Can you work these out from the model? Positions are in its coordinate system, mm. A direction names the side the tool comes from. Coordinates: 2 decimals unless noted, no trailing zeros. Order: outer loops, then holes, each group sorted by start corner. A loop starts at its lowest first (then second) coordinate and runs counter-clockwise, first axis right, second up.
```python
from build123d import *

# Parameters (mm, degrees)
SKETCH1_W              = 220
SKETCH1_H              = 90
SKETCH1_R              = 3
SKETCH1_R_2            = 5.25
BOSS_EXTRUDE1_DEPTH    = 4
SKETCH3_W              = 4
SKETCH3_H              = 90
BOSS_EXTRUDE2_DEPTH    = 10
SKETCH21_W             = 220
SKETCH21_H             = 90
SKETCH21_R             = 5.25
SKETCH21_R_2           = 10
SKETCH21_R_3           = 5
BOSS_EXTRUDE3_DEPTH    = 4
CUT_EXTRUDE4_REACH     = 240.109
SKETCH35_R             = 5
BOSS_EXTRUDE6_DEPTH    = 4
SKETCH33_W             = 1
SKETCH33_H             = 43.95
CUT_EXTRUDE2_DEPTH     = 4
CUT_EXTRUDE3_DEPTH     = 4
SKETCH41_W             = 4
SKETCH41_H             = 16
BOSS_EXTRUDE8_DEPTH    = 26
CONVERT_SOLID4_DEPTH   = 90
CONVERT_SOLID4_START   = 13
CONVERT_SOLID4_2_DEPTH = 20
CONVERT_SOLID4_3_DEPTH = 2
CONVERT_SOLID4_START_2 = 31
CONVERT_SOLID4_4_DEPTH = 2
CONVERT_SOLID4_5_DEPTH = 90
CONVERT_SOLID4_START_3 = 15
CONVERT_SOLID4_6_DEPTH = 16


# Read off the part's stored shape, not the designer's step: Convert-Solid4
with BuildPart() as part:
    # Sketch1 → Boss-Extrude1 (new body)
    with BuildSketch(Plane.XY):
        with Locations((110, 45)):
            Rectangle(SKETCH1_W, SKETCH1_H)
        with Locations((201, 44.75)):
            Circle(SKETCH1_R, mode=Mode.SUBTRACT)
        with Locations((201, 77.75)):
            Circle(SKETCH1_R_2, mode=Mode.SUBTRACT)
        with Locations((15, 44.75)):
            Circle(SKETCH1_R, mode=Mode.SUBTRACT)
        with Locations((15, 77.75)):
            Circle(SKETCH1_R_2, mode=Mode.SUBTRACT)
    extrude(amount=BOSS_EXTRUDE1_DEPTH)

    # Sketch3 → Boss-Extrude2 (add)
    with BuildSketch(Plane.XY.offset(4)):
        with Locations((2, 45)):
            Rectangle(SKETCH3_W, SKETCH3_H)
        with Locations((218, 45)):
            Rectangle(SKETCH3_W, SKETCH3_H)
    extrude(amount=BOSS_EXTRUDE2_DEPTH)

    # Sketch21 → Boss-Extrude3 (add)
    with BuildSketch(Plane.XY.offset(14)):
        with Locations((110, 45)):
            Rectangle(SKETCH21_W, SKETCH21_H)
        with Locations((201, 77.75)):
            Circle(SKETCH21_R, mode=Mode.SUBTRACT)
        with Locations((15, 77.75)):
            Circle(SKETCH21_R, mode=Mode.SUBTRACT)
        with Locations((15, 44.75)):
            Circle(SKETCH21_R_2, mode=Mode.SUBTRACT)
        with Locations((201, 44.75)):
            Circle(SKETCH21_R_2, mode=Mode.SUBTRACT)
        with Locations((100, 20)):
            Circle(SKETCH21_R_3, mode=Mode.SUBTRACT)
        with Locations((173.090932683, 46.602923891)):
            Circle(SKETCH21_R_3, mode=Mode.SUBTRACT)
        with Locations((155, 75)):
            Circle(SKETCH21_R_3, mode=Mode.SUBTRACT)
    extrude(amount=BOSS_EXTRUDE3_DEPTH)

    # Sketch35 → Cut-Extrude4 (cut, up to next)
    with BuildSketch(Plane.XY.offset(4), mode=Mode.PRIVATE) as cut_extrude4_sk1:
        with Locations((100, 20)):
            Circle(SKETCH35_R)
    cut_extrude4_tool1 = extrude(cut_extrude4_sk1.sketch, amount=-CUT_EXTRUDE4_REACH, mode=Mode.PRIVATE) & part.part
    # Sketch35 → Cut-Extrude4 (cut, up to next)
    with BuildSketch(Plane.XY.offset(4), mode=Mode.PRIVATE) as cut_extrude4_sk2:
        with Locations((173.090932683, 46.602923891)):
            Circle(SKETCH35_R)
    cut_extrude4_tool2 = extrude(cut_extrude4_sk2.sketch, amount=-CUT_EXTRUDE4_REACH, mode=Mode.PRIVATE) & part.part
    # Sketch35 → Cut-Extrude4 (cut, up to next)
    with BuildSketch(Plane.XY.offset(4), mode=Mode.PRIVATE) as cut_extrude4_sk3:
        with Locations((155, 75)):
            Circle(SKETCH35_R)
    cut_extrude4_tool3 = extrude(cut_extrude4_sk3.sketch, amount=-CUT_EXTRUDE4_REACH, mode=Mode.PRIVATE) & part.part
    add(cut_extrude4_tool1.solids().sort_by_distance((100, 20, 4))[0], mode=Mode.SUBTRACT)
    add(cut_extrude4_tool2.solids().sort_by_distance((173.090933, 46.602924, 4))[0], mode=Mode.SUBTRACT)
    add(cut_extrude4_tool3.solids().sort_by_distance((155, 75, 4))[0], mode=Mode.SUBTRACT)

    # Sketch24 → Boss-Extrude6 (add)
    with BuildSketch(Plane(origin=(220, 0, 0), x_dir=(0, 0, -1), z_dir=(1, 0, 0))):
        with BuildLine():
            Line((40, 42.05), (40, 46.05))
            Line((40, 46.05), (0, 46.05))
            Line((0, 46.05), (0, 0))
            Line((0, 0), (40, 0))
            Line((40, 0), (40, 3.95))
            Line((40, 3.95), (35, 3.95))
            ThreePointArc((35, 3.95), (25.715537172, 6.365660518), (18.785731592, 13))
            Line((18.785731592, 13), (15.95, 13))
            Line((15.95, 13), (15.95, 33))
            Line((15.95, 33), (18.785731592, 33))
            ThreePointArc((18.785731592, 33), (25.715537172, 39.634339482), (35, 42.05))
            Line((35, 42.05), (40, 42.05))
        make_face()
    extrude(amount=-BOSS_EXTRUDE6_DEPTH)

    # Sketch33 → Cut-Extrude2 (cut)
    with BuildSketch(Plane(origin=(220, 0, 0), x_dir=(0, 0, -1), z_dir=(1, 0, 0))):
        with Locations((-4.5, 68.025)):
            Rectangle(SKETCH33_W, SKETCH33_H)
    extrude(amount=-CUT_EXTRUDE2_DEPTH, mode=Mode.SUBTRACT)

    # Sketch34 → Cut-Extrude3 (cut)
    with BuildSketch(Plane(origin=(0, 0, 0), x_dir=(-1, 0, 0), z_dir=(0, 0, -1))):
        Polygon((-216, 0), (-215, 0), (-215, 47.05), (-220, 47.05), (-220, 46.05), (-216, 46.05), align=None)
    extrude(amount=-CUT_EXTRUDE3_DEPTH, mode=Mode.SUBTRACT)

    # Sketch41 → Boss-Extrude8 (add)
    with BuildSketch(Plane(origin=(220, 0, 0), x_dir=(0, 0, -1), z_dir=(1, 0, 0))):
        with Locations((13.95, 23)):
            Rectangle(SKETCH41_W, SKETCH41_H)
    extrude(amount=BOSS_EXTRUDE8_DEPTH)

    # Convert-Solid4 outline → Convert-Solid4 (cut)
    with BuildSketch(Plane(origin=(0, 0, 0), x_dir=(1, 0, 0), z_dir=(0, 1, 0))):
        with BuildLine():
            Line((220, 15.95), (220, 15.848979486))
            ThreePointArc((220, 15.848979486), (220.49745519, 15.924680765), (221, 15.95))
            Line((221, 15.95), (220, 15.95))
        make_face()
        with BuildLine():
            ThreePointArc((0, -5), (1.464466094, -1.464466094), (5, 0))
            Line((5, 0), (0, 0))
            Line((0, 0), (0, -5))
        make_face()
        with BuildLine():
            Line((220, -18), (220, -13))
            ThreePointArc((220, -13), (218.535533906, -16.535533906), (215, -18))
            Line((215, -18), (220, -18))
        make_face()
        with BuildLine():
            ThreePointArc((5, -18), (1.464466094, -16.535533906), (0, -13))
            Line((0, -13), (0, -18))
            Line((0, -18), (5, -18))
        make_face()
    extrude(amount=CONVERT_SOLID4_DEPTH, mode=Mode.SUBTRACT)

    # Convert-Solid4 2 outline → Convert-Solid4 2 (cut)
    with BuildSketch(Plane(origin=(0, 0, 0), x_dir=(1, 0, 0), z_dir=(0, 1, 0)).offset(CONVERT_SOLID4_START)):
        with BuildLine():
            Line((216, 15.95), (216, 10.95))
            ThreePointArc((216, 10.95), (217.127016654, 14.11227766), (220, 15.848979486))
            Line((220, 15.848979486), (220, 15.95))
            Line((220, 15.95), (216, 15.95))
        make_face()
    extrude(amount=CONVERT_SOLID4_2_DEPTH, mode=Mode.SUBTRACT)

    # Convert-Solid4 3 outline → Convert-Solid4 3 (cut)
    with BuildSketch(Plane(origin=(0, 0, 0), x_dir=(1, 0, 0), z_dir=(0, 1, 0)).offset(CONVERT_SOLID4_START)):
        with BuildLine():
            Line((216, 10.95), (216, 4.95))
            Line((216, 4.95), (220, 4.95))
            Line((220, 4.95), (220, 15.848979486))
            ThreePointArc((220, 15.848979486), (217.127016654, 14.11227766), (216, 10.95))
        make_face()
    extrude(amount=CONVERT_SOLID4_3_DEPTH, mode=Mode.SUBTRACT)

    # Convert-Solid4 4 outline → Convert-Solid4 4 (cut)
    with BuildSketch(Plane(origin=(0, 0, 0), x_dir=(1, 0, 0), z_dir=(0, 1, 0)).offset(CONVERT_SOLID4_START_2)):
        with BuildLine():
            Line((216, 10.95), (216, 4.95))
            Line((216, 4.95), (220, 4.95))
            Line((220, 4.95), (220, 15.848979486))
            ThreePointArc((220, 15.848979486), (217.127016654, 14.11227766), (216, 10.95))
        make_face()
    extrude(amount=CONVERT_SOLID4_4_DEPTH, mode=Mode.SUBTRACT)

    # Convert-Solid4 5 outline → Convert-Solid4 5 (add)
    with BuildSketch(Plane(origin=(0, 0, 0), x_dir=(1, 0, 0), z_dir=(0, 1, 0))):
        with BuildLine():
            Line((216, -14), (216, -13))
            ThreePointArc((216, -13), (215.707106781, -13.707106781), (215, -14))
            Line((215, -14), (216, -14))
        make_face()
        with BuildLine():
            ThreePointArc((4, -5), (4.292893219, -4.292893219), (5, -4))
            Line((5, -4), (4, -4))
            Line((4, -4), (4, -5))
        make_face()
        with BuildLine():
            Line((4, -14), (5, -14))
            ThreePointArc((5, -14), (4.292893219, -13.707106781), (4, -13))
            Line((4, -13), (4, -14))
        make_face()
    extrude(amount=CONVERT_SOLID4_5_DEPTH)

    # Convert-Solid4 6 outline → Convert-Solid4 6 (add)
    with BuildSketch(Plane(origin=(0, 0, 0), x_dir=(1, 0, 0), z_dir=(0, 1, 0)).offset(CONVERT_SOLID4_START_3)):
        with BuildLine():
            Line((220, 11.95), (220, 10.95))
            ThreePointArc((220, 10.95), (220.292893219, 11.657106781), (221, 11.95))
            Line((221, 11.95), (220, 11.95))
        make_face()
    extrude(amount=CONVERT_SOLID4_6_DEPTH)


solid = part.part
```
1. On a 3-axis mill with a long thin cutter (end or side, diameter ignored), from which of +Z, -Z, +X, -X, +Y, -Y can I reach the whole of each face in a straight line? I mean faces 1 (the cylindrical face through (219, 44, 16)), 2 (the cylindrical face through (151, 72, 2)), 3 (the flat face through (109, 46, 14)), 4 (the cylindrical face through (12.83, 34.99, 15.97)), 5 (the cylindrical face through (218.03, 39.57, -25.6)). Say none if no direction works.
Completed:
face 1: +Z, +X, +Y, -Y
face 2: +Z, -Z
face 3: +Y, -Y
face 4: +Z
face 5: -Z, +X, -X
2. Imagine slicing it at C-C on x = 64. Please give me the cut outline in (y, z), then the cut area to 3 significant figures.
Completed:
outline: (0, 0) - (90, 0) - (90, 4) - (0, 4) - close; (0, 14) - (90, 14) - (90, 18) - (0, 18) - close
area: 720 mm2
3. Imagine slicing it at B-B on y = 20. Please give me the cut outline in (x, z).
Completed:
outline: (0, 5) arc R5 ccw to (5, 0) - (95, 0) - (95, 4) - (5, 4) arc R1 cw to (4, 5) - (4, 13) arc R1 cw to (5, 14) - (95, 14) - (95, 18) - (5, 18) arc R5 ccw to (0, 13) - close; (105, 0) - (215, 0) - (215, 4) - (105, 4) - close; (105, 14) - (215, 14) arc R1 cw to (216, 13) - (216, -10.95) arc R5 ccw to (221, -15.95) - (246, -15.95) - (246, -11.95) - (221, -11.95) arc R1 cw to (220, -10.95) - (220, 13) arc R5 ccw to (215, 18) - (105, 18) - close
4. Thinking about a two-plate mould opening in Y: for faces 6 (the cylindrical face through (104.619, 18.085, 2.028)), 7 (the flat face through (108, 90, 15)), 8 (the cylindrical face through (2, 44, 17)), which applies, pulls with the +Y half, pulls with the -Y half, needs draft (parallel to the pull), parting line crosses it, or undercut?
Completed:
face 6: undercut
face 7: pulls with the +Y half
face 8: needs draft
5. I'm going to push flat-ended pins straight in: pin 1 (5 mm diameter, centred on x = 15, y = 44.75, fed in from -Z); pin 2 (4.5 mm diameter, centred on x = 218.5, y = 59.5, fed in from -Z); pin 3 (3 mm diameter, centred on x = 218.5, z = -22.5, fed in from +Y); pin 4 (5 mm diameter, centred on x = 228, y = 20, fed in from -Z). Where does each tip first touch, or does it pass through?
Completed:
pin 1: passes through
pin 2: stops at z = 0
pin 3: stops at y = 46.05
pin 4: stops at z = -15.95
6. Please list where these lines run through material, in increasing order: probe 1 along Y at (x, z) = (201, 15); probe 2 along Z at (x, y) = (98, 52); probe 3 along X at (y, z) = (52, 12.5).
Completed:
probe 1: y = 0 to 34.75, 54.75 to 72.5, 83 to 90
probe 2: z = 0 to 4, 14 to 18
probe 3: x = 0 to 4, 216 to 220
7. Imagine slicing it at D-D on x = 201. Please give me the cut outline in (y, z).
Completed:
outline: (0, 0) - (41.75, 0) - (41.75, 4) - (0, 4) - close; (0, 14) - (34.75, 14) - (34.75, 18) - (0, 18) - close; (47.75, 0) - (72.5, 0) - (72.5, 4) - (47.75, 4) - close; (54.75, 14) - (72.5, 14) - (72.5, 18) - (54.75, 18) - close; (83, 0) - (90, 0) - (90, 4) - (83, 4) - close; (83, 14) - (90, 14) - (90, 18) - (83, 18) - close
8. Imagine slicing it at A-A on x = 100. Please give me the cut outline in (y, z).
Completed:
outline: (0, 0) - (15, 0) - (15, 4) - (0, 4) - close; (0, 14) - (15, 14) - (15, 18) - (0, 18) - close; (25, 0) - (90, 0) - (90, 4) - (25, 4) - close; (25, 14) - (90, 14) - (90, 18) - (25, 18) - close
